```python
from build123d import *

# Parameters (mm, degrees)
Y_KSEKLIK_EKSTR_ZYON1_DEPTH = 37.5
RADYUS1_R                   = 1
Y_KSEKLIK_EKSTR_ZYON3_DEPTH = 2.5
KES_EKSTR_ZYON1_DEPTH       = 1.6
IZIM4_R                     = 6
Y_KSEKLIK_EKSTR_ZYON4_DEPTH = 1
IZIM5_R                     = 5.5
Y_KSEKLIK_EKSTR_ZYON5_DEPTH = 1
IZIM6_R                     = 3
Y_KSEKLIK_EKSTR_ZYON6_DEPTH = 4


with BuildPart() as part:
    # Çizim1 → Yükseklik-Ekstrüzyon1 (new body)
    with BuildSketch(Plane(origin=(0, 0, 0), x_dir=(1, 0, 0), z_dir=(0, 1, 0))):
        with BuildLine():
            Line((1, 0), (39, 0))
            ThreePointArc((39, 0), (39.707106781, 0.292893219), (40, 1))
            Line((40, 1), (40, 19))
            ThreePointArc((40, 19), (39.707106781, 19.707106781), (39, 20))
            Line((39, 20), (1, 20))
            ThreePointArc((1, 20), (0.292893219, 19.707106781), (0, 19))
            Line((0, 19), (0, 1))
            ThreePointArc((0, 1), (0.292893219, 0.292893219), (1, 0))
        make_face()
    extrude(amount=Y_KSEKLIK_EKSTR_ZYON1_DEPTH)

    # Radyus1
    radyus1_edges = [part.edges().sort_by_distance(p)[0] for p in [
        (0.292893219, 37.5, -19.707106781),
        (0, 37.5, -10),
        (0.292893219, 37.5, -0.292893219),
        (20, 37.5, 0),
        (39.707106781, 37.5, -0.292893219),
        (40, 37.5, -10),
        (39.707106781, 37.5, -19.707106781),
        (20, 37.5, -20),
    ]]
    fillet(radyus1_edges, radius=RADYUS1_R)

    # Çizim2 → Yükseklik-Ekstrüzyon3 (add)
    with BuildSketch(Plane(origin=(0, 10.5, 0), x_dir=(1, 0, 0), z_dir=(0, 1, 0))):
        with BuildLine():
            Line((-5.732050808, 4), (-6, 4))
            Line((-6, 4), (-6, 2.25))
            ThreePointArc((-6, 2.25), (-5.707106781, 1.542893219), (-5, 1.25))
            Line((-5, 1.25), (0, 1.25))
            Line((0, 1.25), (0, 18.75))
            Line((0, 18.75), (-5, 18.75))
            ThreePointArc((-5, 18.75), (-5.707106781, 18.457106781), (-6, 17.75))
            Line((-6, 17.75), (-6, 16))
            Line((-6, 16), (-5.732050808, 16))
            ThreePointArc((-5.732050808, 16), (-2, 15), (-5.732050808, 14))
            Line((-5.732050808, 14), (-6, 14))
            Line((-6, 14), (-6, 6))
            Line((-6, 6), (-5.732050808, 6))
            ThreePointArc((-5.732050808, 6), (-2, 5), (-5.732050808, 4))
        make_face()
        with BuildLine():
            Line((40, 1.25), (45, 1.25))
            ThreePointArc((45, 1.25), (45.707106781, 1.542893219), (46, 2.25))
            Line((46, 2.25), (46, 4))
            Line((46, 4), (45.732050808, 4))
            ThreePointArc((45.732050808, 4), (42, 5), (45.732050808, 6))
            Line((45.732050808, 6), (46, 6))
            Line((46, 6), (46, 14))
            Line((46, 14), (45.732050808, 14))
            ThreePointArc((45.732050808, 14), (42, 15), (45.732050808, 16))
            Line((45.732050808, 16), (46, 16))
            Line((46, 16), (46, 17.75))
            ThreePointArc((46, 17.75), (45.707106781, 18.457106781), (45, 18.75))
            Line((45, 18.75), (40, 18.75))
            Line((40, 18.75), (40, 1.25))
        make_face()
    extrude(amount=-Y_KSEKLIK_EKSTR_ZYON3_DEPTH)

    # Çizim3 → Kes-Ekstrüzyon1 (cut)
    with BuildSketch(Plane.XZ):
        with BuildLine():
            Line((6, -0.5), (26.877501001, -0.5))
            ThreePointArc((26.877501001, -0.5), (28.418861192, -0.125791167), (30.000000044, 0))
            Line((30.000000044, 0), (1, 0))
            ThreePointArc((1, 0), (0.292893219, -0.292893219), (0, -1))
            Line((0, -1), (0, -19))
            ThreePointArc((0, -19), (0.292893219, -19.707106781), (1, -20))
            Line((1, -20), (30.000000006, -20))
            ThreePointArc((30.000000006, -20), (28.418861173, -19.87420883), (26.877501001, -19.5))
            Line((26.877501001, -19.5), (6, -19.5))
            Line((6, -19.5), (6, -14))
            ThreePointArc((6, -14), (4.744562647, -10), (6, -6))
            Line((6, -6), (6, -0.5))
        make_face()
        with BuildLine():
            Line((40, -19), (40, -10))
            ThreePointArc((40, -10), (37.071067814, -17.07106781), (30.000000006, -20))
            Line((30.000000006, -20), (39, -20))
            ThreePointArc((39, -20), (39.707106781, -19.707106781), (40, -19))
        make_face()
        with BuildLine():
            Line((39, 0), (30.000000044, 0))
            ThreePointArc((30.000000044, 0), (37.071067828, -2.928932204), (40, -10))
            Line((40, -10), (40, -1))
            ThreePointArc((40, -1), (39.707106781, -0.292893219), (39, 0))
        make_face()
    extrude(amount=-KES_EKSTR_ZYON1_DEPTH, mode=Mode.SUBTRACT)

    # Çizim4 → Yükseklik-Ekstrüzyon4 (add)
    with BuildSketch(Plane.XZ):
        with Locations(Location((30, -10, 0), (0, 0, 90))):
            Circle(IZIM4_R)
    extrude(amount=Y_KSEKLIK_EKSTR_ZYON4_DEPTH)

    # Çizim5 → Yükseklik-Ekstrüzyon5 (add)
    with BuildSketch(Plane.XZ.offset(1)):
        with Locations(Location((30, -10, 0), (0, 0, 270))):
            Circle(IZIM5_R)
    extrude(amount=Y_KSEKLIK_EKSTR_ZYON5_DEPTH)

    # Çizim6 → Yükseklik-Ekstrüzyon6 (add)
    with BuildSketch(Plane.XZ.offset(2)):
        with Locations(Location((30, -10, 0), (0, 0, 270))):
            Circle(IZIM6_R)
    extrude(amount=Y_KSEKLIK_EKSTR_ZYON6_DEPTH)


solid = part.part
```
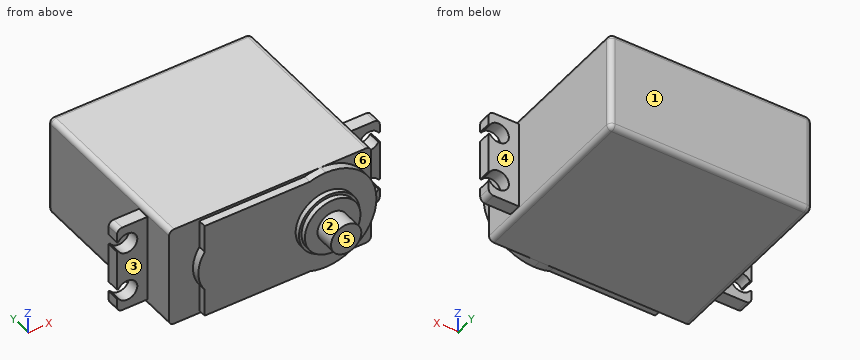
Here's how the part is built. I have some questions about the finished solid (model axes, mm). Face numbers are marked on the shaded views. A direction names the side the tool comes from. Coordinates: 2 decimals unless noted, no trailing zeros. Order: outer loops, then holes, each group sorted by start corner. A loop starts at its lowest first (then second) coordinate and runs counter-clockwise, first axis right, second up. Notation, with made-up numbers: (-8, 17.5) - (1, 17.5) arc R10 ccw to (1, 21.5) - close; hole circle Ø9 at (13, 44). An arc over 180 degrees is marked (long way). One line per question, with ' | ' between items.
(1) Suppose I cut it at C-C on x = 12. List the corners of the cut face in (y, z) for me, and give its area (3 significant figures).
Report:
outline: (0, -19.5) - (1.6, -19.5) - (1.6, -20) - (36.5, -20) arc R1 ccw to (37.5, -19) - (37.5, -1) arc R1 ccw to (36.5, 0) - (1.6, 0) - (1.6, -0.5) - (0, -0.5) - close | area: 748 mm2
(2) If I drill on L1, parallel to Z at x = -4, y = 9; L2, parallel to X at y = 15.5, z = -18.5; L3, parallel to X at y = 8.85, z = -15, over which ranges is the centre line in solid material (lowest first)?
Report:
L1: z = -18.75 to -17, -13 to -7, -3 to -1.25 | L2: x = 0 to 40 | L3: x = -2 to 42
(3) For the marked faces 3, 4, 5 and 6, which set-ups out of +Z, -Z, +X, -X, +Y, -Y let a thin tool reach every point of the face, with its end or its side?
Report:
face 3: +Z, -Z, -X, -Y | face 4: +Z, -Z, +X, +Y | face 5: +Z, -Z, +X, -X, -Y | face 6: +Z, +X, -Y
(4) Will these pins go through, and if not, where does the flat tip stop? pin 1 (2.5 mm diameter, centred on x = 44, z = -15, fed in from -Y); pin 2 (1 mm diameter, centred on x = 13, z = -4, fed in from -Y); pin 3 (3 mm diameter, centred on x = -2, y = 9.5, fed in from +Z); pin 4 (8 mm diameter, centred on y = 16, z = -9, fed in from -X).
Report:
pin 1: passes through | pin 2: stops at y = 0 | pin 3: stops at z = -1.25 | pin 4: stops at x = 0
(5) Suppose I cut it at B-B on y = 22. List the corners of the cut face in (x, z) for me, and give its area (3 significant figures).
Report:
outline: (0, -19) arc R1 ccw to (1, -20) - (39, -20) arc R1 ccw to (40, -19) - (40, -1) arc R1 ccw to (39, 0) - (1, 0) arc R1 ccw to (0, -1) - close | area: 799 mm2
(6) Suppose I cut it at A-A on x = -4. List the corners of the cut face in (y, z) for me.
Report:
outline: (8, -18.75) - (10.5, -18.75) - (10.5, -17) - (8, -17) - close; (8, -13) - (10.5, -13) - (10.5, -7) - (8, -7) - close; (8, -3) - (10.5, -3) - (10.5, -1.25) - (8, -1.25) - close
(7) If we mould it in two halves opening along X, with no side actions, what happens to the marked faces 1 and 2? For each: pulls with the +X half, pulls with the -X half, needs draft (parallel to the pull), parting line crosses it, or undercut.
Report:
face 1: needs draft | face 2: parting line crosses it
